Could you check a few things on this model? Use its own coordinates, in mm. Face numbers are marked on the shaded views. Give positions to 0.01 mm unless a question says otherwise; leave off trailing zeros. Order: outer loops, then holes, each group sorted by start corner. A loop starts at its lowest first (then second) coordinate and runs counter-clockwise, first axis right, second up.
(1) Will these pins go through, and if not, where does the flat tip stop? pin 1 (3 mm diameter, centred on y = 6.5, z = 6, fed in from +X); pin 2 (3 mm diameter, centred on x = -51, z = 11, fed in from -Y); pin 3 (2 mm diameter, centred on x = -24.5, z = 7.5, fed in from +Y).
(2) Imagine slicing it at B-B, the plane z = 5. Write out the boundary of the cut face in (x, y), then the cut area to 3 significant figures.
(3) If I drill on probe 1 along X at (y, z) = (-15.5, -3); probe 2 along Y at (x, z) = (-50, -5); probe 3 along X at (y, z) = (-28, 17.5), over which ranges is the centre line in solid material (lowest first)?
(4) Imagine slicing it at A-A, the plane z = 17.5. Write out the boundary of the cut face in (x, y), then the cut area to 3 significant figures.
(5) If we mould it in two halves opening along X, with no side actions, what happens to the marked faces 1, 2 and 3? For each: released by +X, released by -X, zero draft, split by the parting line, or undercut.
from build123d import *

# Parameters (mm, degrees)
F0_W     = 48.2568442822
F0_H     = 32.1138165891
F1_DEPTH = 28.194
F2_SIZE  = 20.32
F4_R     = 18.934689064
F5_DEPTH = 32.1138165891


with BuildPart() as f1:
    # F0 (on Front) → F1 (new body)
    with BuildSketch(Plane.XZ):
        with Locations((-83.3175331354, 7.1921925992)):
            Rectangle(F0_W, F0_H)
    extrude(amount=F1_DEPTH)

    # F2
    f2_edges = [f1.edges().sort_by_distance(p)[0] for p in [
        (-107.445955, -14.097, 23.249101),
    ]]
    chamfer(f2_edges, length=F2_SIZE)

    # F1_face (on face) → F3 (revolve)
    with BuildSketch(Plane(origin=(-80.6501580531, -28.194, 5.7653617255), x_dir=(1, 0, 0), z_dir=(0, -1, 0))):
        Polygon((21.4610470587, 17.4837391683), (-6.4757972234, 17.4837391683), (-26.7957972234, -2.8362608317), (-26.7957972234, -14.6300774209), (21.4610470587, -14.6300774209), align=None)
    revolve(axis=Axis((-59.1891109943, -28.194, 7.1921925992), (0, 0, -1)))

    # F4 (on face) → F5 (cut, through all)
    with BuildSketch(Plane.XY.offset(23.2491008937)):
        with Locations((-59.1891109943, -28.194)):
            Circle(F4_R)
    extrude(amount=-F5_DEPTH, mode=Mode.SUBTRACT)


solid = f1.part
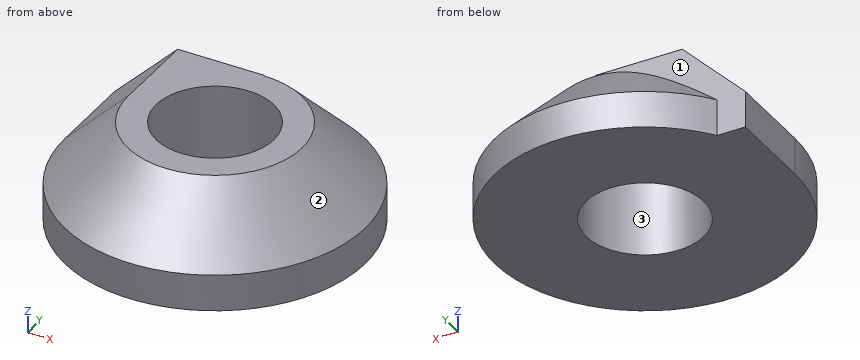
Answer block:
1. pin 1: stops at x = -27.41
1. pin 2: stops at y = -69.1
1. pin 3: stops at y = 0.39
2. outline: (-105.38, -28.19) arc R46.19 ccw (long way) to (-95.77, 0) - (-105.38, 0) - close; hole circle Ø37.87 at (-59.19, -28.19)
2. area: 5,660 mm2
3. probe 1: x = -107.45 to -73.24, -45.14 to -12.63
3. probe 2: y = -75.57 to -44.75, -11.64 to 19.18
3. probe 3: x = -92.88 to -78.12, -40.26 to -25.5
4. outline: (-92.88, -28.19) arc R33.69 ccw (long way) to (-77.62, 0) - (-92.88, 0) - close; hole circle Ø37.87 at (-59.19, -28.19)
4. area: 2,570 mm2
5. face 1: zero draft
5. face 2: split by the parting line
5. face 3: undercut
